```python
from build123d import *

# Parameters (mm, degrees)
SKETCH2_W           = 177.5
SKETCH2_H           = 180
BOSS_EXTRUDE1_DEPTH = 3
SKETCH4_W           = 50
SKETCH4_H           = 30
BOSS_EXTRUDE2_DEPTH = 6.5
CUT_EXTRUDE1_DEPTH  = 5
SKETCH6_W           = 44
SKETCH6_H           = 12
CUT_EXTRUDE2_DEPTH  = 6.5
FILLET1_R           = 5
FILLET2_R           = 5


with BuildPart() as part:
    # Sketch2 → Boss-Extrude1 (new body)
    with BuildSketch(Plane.XY):
        with Locations((88.75, 90)):
            Rectangle(SKETCH2_W, SKETCH2_H)
    extrude(amount=-BOSS_EXTRUDE1_DEPTH)

    # Sketch4 → Boss-Extrude2 (add)
    with BuildSketch(Plane.XY.offset(-1.5)):
        with Locations((90, 180)):
            Rectangle(SKETCH4_W, SKETCH4_H)
    extrude(amount=-BOSS_EXTRUDE2_DEPTH)

    # Sketch5 → Cut-Extrude1 (cut)
    with BuildSketch(Plane(origin=(0, 0, -8), x_dir=(-1, 0, 0), z_dir=(0, 0, -1))):
        Polygon((-112, 168), (-112, 165), (-68, 165), (-68, 168), (-68, 192), (-112, 192), align=None)
    extrude(amount=-CUT_EXTRUDE1_DEPTH, mode=Mode.SUBTRACT)

    # Sketch6 → Cut-Extrude2 (cut)
    with BuildSketch(Plane.XY.offset(-1.5)):
        with Locations((90, 186)):
            Rectangle(SKETCH6_W, SKETCH6_H)
    extrude(amount=-CUT_EXTRUDE2_DEPTH, mode=Mode.SUBTRACT)

    # Fillet1
    fillet1_edges = [part.edges().sort_by_distance(p)[0] for p in [
        (115, 195, -4.75),
    ]]
    fillet(fillet1_edges, radius=FILLET1_R)

    # Fillet2
    fillet2_edges = [part.edges().sort_by_distance(p)[0] for p in [
        (65, 195, -4.75),
    ]]
    fillet(fillet2_edges, radius=FILLET2_R)


solid = part.part
```
The model under review builds one solid part; all positions refer to its coordinate system, in mm. A direction names the side the tool comes from. Give positions to 0.01 mm unless a question says otherwise; leave off trailing zeros. Loops run counter-clockwise (first coordinate to the right, second up) from the corner with the lowest first, then second, coordinate; pieces in that order, holes last. Notation, with made-up numbers: (48, 14.25) - (71, 14.25) arc R19 ccw to (71, 39.25) - close; hole circle Ø11 at (44.5, -38.75). An arc over 180 degrees is marked (long way). Answer as a JSON object with one key per item and string values.
Q1. Add section C-C on y = 145.5. State the section outline as (x, z) points, plus the area to 4 significant figures.
Worked out:
{"outline": "(0, -3) - (177.5, -3) - (177.5, 0) - (0, 0) - close", "area": "532.5 mm^2"}
Q2. Mouldability with a two-part tool opening along X and no side actions: class faces 1 (the cylindrical face through (114, 193, -5)), 2 (the cylindrical face through (67, 194, -5)), 3 (the flat face through (90, 192, -5)) as +X half, -X half, draft (parallel to the pull), parting line (faces both ways), or undercut.
Worked out:
{"face 1": "+X half", "face 2": "-X half", "face 3": "undercut"}
Q3. For faces 4 (the flat face through (90, 193, -1.5)), 5 (the flat face through (90, 195, -5)), list the 3-axis set-ups (+Z, -Z, +X, -X, +Y, -Y) from which the entire face can be reached by the end or side of a thin tool; tool diameter is ignored.
Worked out:
{"face 4": "+Z, +X, -X, +Y", "face 5": "+Z, -Z, +X, -X, +Y"}
Q4. Insertion check: pin 1 (1.5 mm diameter, centred on x = 66, z = -4.5, fed in from -Y); pin 2 (2 mm diameter, centred on x = 38, z = -1, fed in from +Y); pin 3 (2 mm diameter, centred on y = 177.5, z = -6, fed in from +X). Each pin has a flat end and moves straight along its axis. Give the tip position at first contact, or say it passes through.
Worked out:
{"pin 1": "stops at y = 165", "pin 2": "stops at y = 180", "pin 3": "stops at x = 115"}
Q5. Add section A-A on x = 75. State the section outline as (y, z) points, plus the area to 4 significant figures.
Worked out:
{"outline": "(0, -3) - (180, -3) - (180, 0) - (0, 0) - close; (192, -8) - (195, -8) - (195, -1.5) - (192, -1.5) - close", "area": "559.5 mm^2"}
Q6. To check wall thickness, follow line 1 along X through (y, z) = (185, -7.5); line 2 along Z through (x, y) = (40.5, 145.5); line 3 along Y through (x, z) = (26, -1.75). State the ranges of each line that lie inside material, in increasing order.
Worked out:
{"line 1": "x = 65 to 68, 112 to 115", "line 2": "z = -3 to 0", "line 3": "y = 0 to 180"}
Q7. Add section D-D on x = 22.5. State the section outline as (y, z) points.
Worked out:
{"outline": "(0, -3) - (180, -3) - (180, 0) - (0, 0) - close"}
Q8. Add section B-B on z = -5.25. State the section outline as (x, y) points.
Worked out:
{"outline": "(65, 165) - (68, 165) - (68, 192) - (112, 192) - (112, 165) - (115, 165) - (115, 190) arc R5 ccw to (110, 195) - (70, 195) arc R5 ccw to (65, 190) - close"}
